Verification items for the finished model (mm, model axes). Face numbers are marked on the shaded views. A direction names the side the tool comes from. Round coordinates to 2 decimals unless told otherwise and drop trailing zeros. Loops run counter-clockwise (first coordinate to the right, second up) from the corner with the lowest first, then second, coordinate; pieces in that order, holes last. Notation, with made-up numbers: M 47,70.25 L 72,70.25 A13 cw 72,83.25 Z; hole C 71,28.25 d4. An arc over 180 degrees is marked long. Answer as CSV lines item,"result".
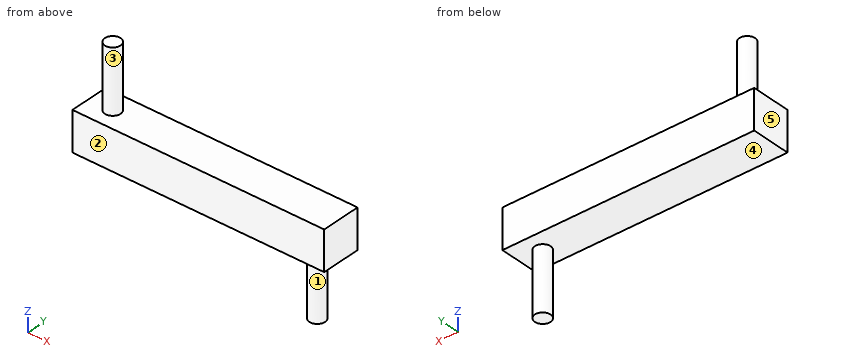
```python
from build123d import *

# Parameters (mm, degrees)
SKETCH1_W           = 16
SKETCH1_H           = 2.5
BOSS_EXTRUDE1_DEPTH = 1.25
SKETCH2_R           = 0.5
BOSS_EXTRUDE2_DEPTH = 4
SKETCH3_R           = 0.5
BOSS_EXTRUDE3_DEPTH = 4


with BuildPart() as part:
    # Sketch1 → Boss-Extrude1 (new body, symmetric)
    with BuildSketch(Plane.XY):
        with Locations((8, 1.25)):
            Rectangle(SKETCH1_W, SKETCH1_H)
    extrude(amount=BOSS_EXTRUDE1_DEPTH, both=True)

    # Sketch2 → Boss-Extrude2 (add)
    with BuildSketch(Plane.XY.offset(1.25)):
        with Locations((1.5, 1.25)):
            Circle(SKETCH2_R)
    extrude(amount=BOSS_EXTRUDE2_DEPTH)

    # Sketch3 → Boss-Extrude3 (add)
    with BuildSketch(Plane(origin=(0, 0, -1.25), x_dir=(-1, 0, 0), z_dir=(0, 0, -1))):
        with Locations((-14.5, 1.25)):
            Circle(SKETCH3_R)
    extrude(amount=BOSS_EXTRUDE3_DEPTH)


solid = part.part
```
1) Section check D-D (y = 0.2). Record the cut outline in (x, z), plus the area to 3 significant figures.
Here are the results:
outline,"M 0,-1.25 L 16,-1.25 L 16,1.25 L 0,1.25 Z"
area,"40.0 mm^2"
2) Section check A-A (y = 1.25). Record the cut outline in (x, z).
Here are the results:
outline,"M 0,-1.25 L 14,-1.25 L 14,-5.25 L 15,-5.25 L 15,-1.25 L 16,-1.25 L 16,1.25 L 2,1.25 L 2,5.25 L 1,5.25 L 1,1.25 L 0,1.25 Z"
3) Section check B-B (x = 14.5). Record the cut outline in (y, z), plus the area to 4 significant figures.
Here are the results:
outline,"M 0,-1.25 L 0.75,-1.25 L 0.75,-5.25 L 1.75,-5.25 L 1.75,-1.25 L 2.5,-1.25 L 2.5,1.25 L 0,1.25 Z"
area,"10.25 mm^2"
4) Set-up check for the marked faces 1 and 2: record each of +Z, -Z, +X, -X, +Y, -Y from which the full face is reachable in a straight line by a thin tool's end or side.
Here are the results:
face 1,"-Z"
face 2,"+Z, -Z, +X, -X, -Y"
5) Material ranges on probe 1 along Z at (x, y) = (12, 0.5); probe 2 along X at (y, z) = (1.5, -4), recorded low to high.
Here are the results:
probe 1,"z = -1.25 to 1.25"
probe 2,"x = 14.07 to 14.93"
6) Section check C-C (z = -3). Record the cut outline in (x, y).
Here are the results:
outline,"C 14.5,1.25 d1"
7) Draft check along X on the marked faces 3, 4 and 5. Enter one of: +X half, -X half, draft (parallel to the pull), parting line (faces both ways), or undercut.
Here are the results:
face 3,"parting line"
face 4,"draft"
face 5,"-X half"
8) Go/stop test with a flat-tipped pin: pin 1 (1 mm diameter, centred on x = 2.5, z = -3.5, fed in from +Y). Record where the tip stops, or that it passes through.
Here are the results:
pin 1,"passes through"
